from build123d import *

# Parameters (mm, degrees)
F1_DEPTH = 15
F3_DEPTH = 30


with BuildPart() as f1:
    # F0 (on Top) → F1 (new body)
    with BuildSketch(Plane.XY):
        with BuildLine():
            Line((0, 0), (25, 0))
            ThreePointArc((25, 0), (16.350977, 76.530518), (-9.159795, 149.200499))
            Line((-9.159795, 149.200499), (-21.486737, 140.02049))
            ThreePointArc((-21.486737, 140.02049), (6.680505, 72.684012), (0, 0))
        make_face()
    extrude(amount=F1_DEPTH)

    # F2 (on Right) → F3 (intersect, symmetric)
    with BuildSketch(Plane.YZ):
        with BuildLine():
            ThreePointArc((149.200499, 5.021363), (74.342296, 6.153758), (0, 15))
            Line((0, 15), (0, 0))
            Line((0, 0), (149.200499, 0))
            Line((149.200499, 0), (149.200499, 5.021363))
        make_face()
    extrude(amount=F3_DEPTH, both=True, mode=Mode.INTERSECT)

    # F4: F1 across plane


with BuildPart() as f1_1:
    add(f1.part)
    add(f1.part.mirror(Plane.XZ))

    # F5: F1 across plane


with BuildPart() as f1_2:
    add(f1_1.part)
    add(f1_1.part.mirror(Plane.XY))


solid = f1_2.part
Build history of the part. All positions in model axes, mm. A direction names the side the tool comes from. Give positions to 0.01 mm unless a question says otherwise; leave off trailing zeros. Loops run counter-clockwise (first coordinate to the right, second up) from the corner with the lowest first, then second, coordinate; pieces in that order, holes last. Notation, with made-up numbers: (48, 75) -> (67, 75) arc R20 cw to (67, 82) -> close; hole circle Ø4 at (-1, -21.5). An arc over 180 degrees is marked (long way). Answer in a Markdown table with one row per item.
Item 1: Slice it at C-C on x = 19.5. Write the cut outline in (y, z), plus the area to 3 significant figures.
Findings below:
| item | result |
|---|---|
| outline | (-61.17, -7.16) arc R725 cw to (0, -15) arc R725 cw to (61.17, -7.16) -> (61.17, 7.16) arc R725 cw to (0, 15) arc R725 cw to (-61.17, 7.16) -> close |
| area | 2,600 mm² |
Item 2: Slice it at D-D on y = 69. Write the cut outline in (x, z).
Findings below:
| item | result |
|---|---|
| outline | (7.2, -6.53) -> (17.99, -6.53) -> (17.99, 6.53) -> (7.2, 6.53) -> close |
Item 3: Slice it at A-A on x = -6.5. Write the cut outline in (y, z), plus the area to 3 significant figures.
Findings below:
| item | result |
|---|---|
| outline | (-143.57, -4.84) arc R725 cw to (-115.25, -4.58) -> (-115.25, 4.58) arc R725 cw to (-143.57, 4.84) -> close; (115.25, -4.58) arc R725 cw to (143.57, -4.84) -> (143.57, 4.84) arc R725 cw to (115.25, 4.58) -> close |
| area | 523 mm² |
Item 4: Tool access for faces 1 (the cylindrical face through (8.75, -63.63, 6.95)), 2 (the cylindrical face through (8.75, -63.63, -6.95)), 3 (the cylindrical face through (8.235, -57.42, 0.21)): list every direction of +Z, -Z, +X, -X, +Y, -Y with a clear straight run to the whole face (end or side of a thin tool).
Findings below:
| item | result |
|---|---|
| face 1 | +Z, +X, -X |
| face 2 | -Z, +X, -X |
| face 3 | +Z, -Z, -X |
Item 5: Mould opens along Y. For faces 4 (the flat face through (-15.2, 144.7, 0.1)), 5 (the cylindrical face through (8.235, 57.42, 0.21)), 6 (the flat face through (-15.2, -144.7, 0.1)), 7 (the cylindrical face through (8.75, 63.63, -6.95)) say: pulls with the +Y half, pulls with the -Y half, needs draft (parallel to the pull), parting line crosses it, or undercut.
Findings below:
| item | result |
|---|---|
| face 4 | pulls with the +Y half |
| face 5 | undercut |
| face 6 | pulls with the -Y half |
| face 7 | undercut |
Item 6: Flat gauge pins, fed straight in: P1, Ø5, axis at x = -14, z = -5.5, coming from the -Y side; P2, Ø8, axis at y = -9.5, z = -5, coming from the -X side; P3, Ø10, axis at x = 3, y = -103.5, coming from the +Z side. Where does each tip first touch, or does it go through?
Findings below:
| item | result |
|---|---|
| P1 | stops at y = -147.41 |
| P2 | stops at x = 1.8 |
| P3 | stops at z = 4.94 |
Item 7: Slice it at B-B on z = 1. Write the cut outline in (x, y).
Findings below:
| item | result |
|---|---|
| outline | (-21.49, -140.02) -> (-9.16, -149.2) arc R342.91 ccw to (25, 0) arc R342.91 ccw to (-9.16, 149.2) -> (-21.49, 140.02) arc R151.11 cw to (0, 0) arc R151.11 cw to start |
Item 8: Probe line 1 along Z through (x, y) = (9, -96); line 2 along Y through (x, z) = (-10, -4); line 3 along X through (y, z) = (-25.5, 10.5). List the from-to ranges inside material, lowest first. Write a range as [from, to].
Findings below:
| item | result |
|---|---|
| line 1 | z = [-5.03, 5.03] |
| line 2 | y = [-148.57, -122.08], [122.08, 148.57] |
| line 3 | x = [6.47, 24.05] |
